Verification items for the finished model (mm, model axes). A direction names the side the tool comes from. Give positions to 0.01 mm unless a question says otherwise; leave off trailing zeros. Write each loop counter-clockwise with the first axis right and the second up, starting at its lowest first coordinate (ties: lowest second). Pieces come first, ordered by that corner, then holes. Notation, with made-up numbers: (57.5, 43) -> (82.5, 43) arc R22 cw to (82.5, 66) -> close; hole circle Ø7 at (60.5, -39). An arc over 180 degrees is marked (long way). Answer as CSV lines item,"result". Start each with the question number.
1) Tool access check on faces 5 (the flat face through (0, 35, 66)), 6 (the flat face through (70, 8, 30)). Record the directions out of +Z, -Z, +X, -X, +Y, -Y that give a thin tool (end or side, any length) a straight path to the whole face; none if there is none.
2) Sectioned sample at B-B on z = 48. Record the cut outline in (x, y).
3) Sectioned sample at A-A on x = 0. Record the cut outline in (y, z), and give its area (3 significant figures).
4) Material ranges on L1, parallel to Z at x = -54, y = 11; L2, parallel to X at y = 6.75, z = 16; L3, parallel to Y at x = 0, z = 3.75, recorded low to high.
5) Sectioned sample at D-D on z = 12. Record the cut outline in (x, y).
6) Sectioned sample at C-C on y = 22.5. Record the cut outline in (x, z).
7) Gauge pin test, flat ends, axial feed: pin 1 Ø6 at (x, y) = (-17.5, 55) entering from +Z; pin 2 Ø8 at (y, z) = (53, 8.5) entering from +X; pin 3 Ø17.5 at (y, z) = (47.5, 4) entering from -X. Record the tip position at first contact, or that the pin passes through.
8) Mould release check, pull along X, two halves, no side actions. Record for faces 1 (the cylindrical face through (65.189, 7.888, 4.563)), 2 (the cylindrical face through (-65.189, 7.888, 4.563)), 3 (the cylindrical face through (-1.041, 67.932, 7.888)), 4 (the flat face through (0, 35, 30)): released by +X, released by -X, zero draft, split by the parting line, or undercut.
```python
from build123d import *

# Parameters (mm, degrees)
EXTRUDE_1_DEPTH     = 80
SKETCH_3_R          = 8
EXTRUDE_2_DEPTH     = 16
SKETCH_4_W          = 84.547176069
SKETCH_4_H          = 36
CUT_EXTRUDE_1_DEPTH = 33
SKETCH_5_R          = 8
EXTRUDE_3_DEPTH     = 16


with BuildPart() as part:
    # 草图2 → 凸台-拉伸1 (new body)
    with BuildSketch(Plane.XY):
        with BuildLine():
            Line((-40, 0), (-24, 0))
            ThreePointArc((-24, 0), (0, 24), (24, 0))
            Line((24, 0), (40, 0))
            ThreePointArc((40, 0), (0, 40), (-40, 0))
        make_face()
    extrude(amount=EXTRUDE_1_DEPTH)

    # 草图3 → 凸台-拉伸2 (add)
    with BuildSketch(Plane(origin=(0, 0, 0), x_dir=(1, 0, 0), z_dir=(0, 1, 0))):
        with BuildLine():
            Line((32.951730358, 0), (54, 0))
            ThreePointArc((54, 0), (65.313708499, -4.686291501), (70, -16))
            Line((70, -16), (70, -44))
            ThreePointArc((70, -44), (65.313708499, -55.313708499), (54, -60))
            Line((54, -60), (32.951730358, -60))
            Line((32.951730358, -60), (32.951730358, 0))
        make_face()
        with Locations((54, -16)):
            Circle(SKETCH_3_R, mode=Mode.SUBTRACT)
        with Locations((54, -44)):
            Circle(SKETCH_3_R, mode=Mode.SUBTRACT)
        with BuildLine():
            Line((-32.951730358, -60), (-32.951730358, 0))
            Line((-32.951730358, 0), (-54, 0))
            ThreePointArc((-54, 0), (-65.313708499, -4.686291501), (-70, -16))
            Line((-70, -16), (-70, -44))
            ThreePointArc((-70, -44), (-65.313708499, -55.313708499), (-54, -60))
            Line((-54, -60), (-32.951730358, -60))
        make_face()
        with Locations((-54, -44)):
            Circle(SKETCH_3_R, mode=Mode.SUBTRACT)
        with Locations((-54, -16)):
            Circle(SKETCH_3_R, mode=Mode.SUBTRACT)
    extrude(amount=EXTRUDE_2_DEPTH)

    # 草图4 → 切除-拉伸1 (cut)
    with BuildSketch(Plane(origin=(0, 32, 0), x_dir=(1, 0, 0), z_dir=(0, 1, 0))):
        with Locations((0.989381847, -48)):
            Rectangle(SKETCH_4_W, SKETCH_4_H)
    extrude(amount=CUT_EXTRUDE_1_DEPTH, mode=Mode.SUBTRACT)

    # 草图5 → 凸台-拉伸3 (add)
    with BuildSketch(Plane.XY):
        with BuildLine():
            Line((-16, 60), (-16, 36.66060556))
            Line((-16, 36.66060556), (16, 36.66060556))
            Line((16, 36.66060556), (16, 60))
            ThreePointArc((16, 60), (0, 76), (-16, 60))
        make_face()
        with Locations((0, 60)):
            Circle(SKETCH_5_R, mode=Mode.SUBTRACT)
    extrude(amount=EXTRUDE_3_DEPTH)


solid = part.part
```
Ans:
1,face 5,"+X, -X, +Y"
1,face 6,"+Z, -Z, +X, +Y, -Y"
2,outline,"(-69.49, 0) -> (-60.93, 0) -> (-60.93, 16) -> (-69.49, 16) -> close; (-47.07, 0) -> (-24, 0) arc R24 cw to (24, 0) -> (47.07, 0) -> (47.07, 16) -> (36.66, 16) arc R40 ccw to (24, 32) -> (-24, 32) arc R40 ccw to (-36.66, 16) -> (-47.07, 16) -> close; (60.93, 0) -> (69.49, 0) -> (69.49, 16) -> (60.93, 16) -> close"
3,outline,"(24, 0) -> (52, 0) -> (52, 16) -> (40, 16) -> (40, 30) -> (32, 30) -> (32, 66) -> (40, 66) -> (40, 80) -> (24, 80) -> close; (68, 0) -> (76, 0) -> (76, 16) -> (68, 16) -> close"
3,area,"1,310 mm²"
4,L1,"z = 0 to 8, 24 to 36, 52 to 60"
4,L2,"x = -70 to -62, -46 to -23.03, 23.03 to 46, 62 to 70"
4,L3,"y = 24 to 52, 68 to 76"
5,outline,"(-69.49, 0) -> (-60.93, 0) -> (-60.93, 16) -> (-69.49, 16) -> close; (-47.07, 0) -> (-24, 0) arc R24 cw to (24, 0) -> (47.07, 0) -> (47.07, 16) -> (36.66, 16) arc R40 ccw to (16, 36.66) -> (16, 60) arc R16 ccw to (-16, 60) -> (-16, 36.66) arc R40 ccw to (-36.66, 16) -> (-47.07, 16) -> close; (60.93, 0) -> (69.49, 0) -> (69.49, 16) -> (60.93, 16) -> close; hole circle Ø16 at (0, 60)"
6,outline,"(-33.07, 0) -> (-8.35, 0) -> (-8.35, 80) -> (-33.07, 80) -> close; (8.35, 0) -> (33.07, 0) -> (33.07, 80) -> (8.35, 80) -> close"
7,pin 1,"stops at z = 16"
7,pin 2,"stops at x = 16"
7,pin 3,"stops at x = -16"
8,face 1,"released by +X"
8,face 2,"released by -X"
8,face 3,"undercut"
8,face 4,"zero draft"
